Design review of the part built by this model. Coordinates are the model's own, in mm. A direction names the side the tool comes from. Give positions to 0.01 mm unless a question says otherwise; leave off trailing zeros. Order: outer loops, then holes, each group sorted by start corner. A loop starts at its lowest first (then second) coordinate and runs counter-clockwise, first axis right, second up.
```python
from build123d import *

# Parameters (mm, degrees)
F0_W     = 23
F0_H     = 12
F1_DEPTH = 2
F3_DEPTH = 35
F5_DEPTH = 2


with BuildPart() as f1:
    # F0 (on Top) → F1 (new body)
    with BuildSketch(Plane.XY):
        Polygon((0, 5), (5, 0), (55, 0), (60, 5), (60, 25), (55, 30), (5, 30), (0, 25), align=None)
        with Locations((30, 16.8)):
            Rectangle(F0_W, F0_H, mode=Mode.SUBTRACT)
    extrude(amount=F1_DEPTH)

    # F2 (on face) → F3 (join)
    with BuildSketch(Plane(origin=(0, 0, 0), x_dir=(1, 0, 0), z_dir=(0, 0, -1))):
        with BuildLine():
            Line((61, -27), (61, -4.585786))
            Line((61, -4.585786), (55.414214, 1))
            Line((55.414214, 1), (4.585786, 1))
            Line((4.585786, 1), (-1, -4.585786))
            Line((-1, -4.585786), (-1, -27))
            ThreePointArc((-1, -27), (0.464466, -30.535534), (4, -32))
            Line((4, -32), (56, -32))
            ThreePointArc((56, -32), (59.535534, -30.535534), (61, -27))
        make_face()
        Polygon((5, -30), (0, -25), (0, -5), (5, 0), (55, 0), (60, -5), (60, -25), (55, -30), align=None, mode=Mode.SUBTRACT)
    extrude(amount=-F3_DEPTH)

    # F4 (on face) → F5 (join)
    with BuildSketch(Plane(origin=(0, 32, 0), x_dir=(-1, 0, 0), z_dir=(0, 1, 0))):
        with BuildLine():
            Line((-56, 35), (-30, 35))
            Line((-30, 35), (-30, 103))
            ThreePointArc((-30, 103), (-32, 105), (-30, 107))
            Line((-30, 107), (-30, 115))
            Line((-30, 115), (-31.333763, 115))
            ThreePointArc((-31.333763, 115), (-34.392289, 113.95543), (-36.172876, 111.258169))
            Line((-36.172876, 111.258169), (-56, 35))
        make_face()
        with BuildLine():
            Line((-30, 103), (-30, 35))
            Line((-30, 35), (-4, 35))
            Line((-4, 35), (-23.827124, 111.258169))
            ThreePointArc((-23.827124, 111.258169), (-25.607711, 113.95543), (-28.666237, 115))
            Line((-28.666237, 115), (-30, 115))
            Line((-30, 115), (-30, 107))
            ThreePointArc((-30, 107), (-28.585786, 106.414214), (-28, 105))
            ThreePointArc((-28, 105), (-28.585786, 103.585786), (-30, 103))
        make_face()
    extrude(amount=-F5_DEPTH)


solid = f1.part
```
1. Take a section at B-B (z = 28). State the section outline as (x, y) points.
Recorded:
outline: (-1, 4.59) - (4.59, -1) - (55.41, -1) - (61, 4.59) - (61, 27) arc R5 ccw to (56, 32) - (4, 32) arc R5 ccw to (-1, 27) - close; hole (0, 5) - (5, 0) - (55, 0) - (60, 5) - (60, 25) - (55, 30) - (5, 30) - (0, 25) - close
2. For line 1 along X through (y, z) = (18.5, 33); line 2 along Y through (x, z) = (32, 25.5); line 3 along Z through (x, y) = (29.5, 7.5), list the stretches that pass through material, from the lowest coordinate up.
Recorded:
line 1: x = -1 to 0, 60 to 61
line 2: y = -1 to 0, 30 to 32
line 3: z = 0 to 2
3. For pin 1 (15.5 mm diameter, centred on x = 41, z = 47, fed in from -Y); pin 2 (3 mm diameter, centred on x = 47, y = 23.5, fed in from +Z); pin 3 (8 mm diameter, centred on y = 26.5, z = 76, fed in from +X); pin 4 (1 mm diameter, centred on x = 24.5, y = 20.5, fed in from +Z), all flat-tipped, find the tip position at first contact; note any pin that passes through.
Recorded:
pin 1: stops at y = 30
pin 2: stops at z = 2
pin 3: stops at x = 45.84
pin 4: passes through
4. Take a section at D-D (x = 26.5). State the section outline as (y, z) points, then the cut area to 3 significant figures.
Recorded:
outline: (-1, 0) - (10.8, 0) - (10.8, 2) - (0, 2) - (0, 35) - (-1, 35) - close; (22.8, 0) - (32, 0) - (32, 114.51) - (30, 114.51) - (30, 2) - (22.8, 2) - close
area: 300 mm2
5. Draft analysis for pull direction Y (two halves, no side actions). For faces 1 (the face through (34.36, 31.01, 113.98)), 2 (the face through (30, 32, 46)), 3 (the face through (57, 2, 18)), state which applies: pulls with the +Y half, pulls with the -Y half, needs draft (parallel to the pull), parting line crosses it, or undercut.
Recorded:
face 1: needs draft
face 2: pulls with the +Y half
face 3: undercut
6. Machinability: for faces 4 (the face through (0, 15, 18)), 5 (the face through (-1, 16, 17)), which of the approach directions +Z, -Z, +X, -X, +Y, -Y give a long, thin tool a straight path to every point of the face, cutting with its end or side? Answer none if there is none.
Recorded:
face 4: +Z
face 5: +Z, -Z, -X, +Y, -Y
7. Take a section at C-C (y = 6.5). State the section outline as (x, z) points.
Recorded:
outline: (-1, 0) - (61, 0) - (61, 35) - (60, 35) - (60, 2) - (0, 2) - (0, 35) - (-1, 35) - close
8. Take a section at A-A (y = 12). State the section outline as (x, z) points, then the cut area to 3 significant figures.
Recorded:
outline: (-1, 0) - (18.5, 0) - (18.5, 2) - (0, 2) - (0, 35) - (-1, 35) - close; (41.5, 0) - (61, 0) - (61, 35) - (60, 35) - (60, 2) - (41.5, 2) - close
area: 144 mm2
